Autodesk Inventor part; units mm, degrees
ref_plane "YZ Plane" through (0, 0, 0) normal (1, 0, 0) x (0, 1, 0)
ref_plane "XZ Plane" through (0, 0, 0) normal (0, 1, 0) x (-1, 0, 0)
ref_plane "XY Plane" through (0, 0, 0) normal (0, 0, 1) x (1, 0, 0)
sketch "Sketch4" plane through (0, 0, 0) normal (0, 0, 1) x (1, 0, 0)
  line L0 (0, 0) -> (26.5, 0)
  line L1 (26.5, 0) -> (26.5, 20.75)
  line L2 (0, 20.75) -> (0, 0)
  arc A0 (26.5, 20.75) -> (0, 20.75) centre (13.25, 20.75) ccw
  line L3 (-1.1061, 34) -> (25.3939, 34) construction
  dimension "d70" = 26.5
  dimension "d71" = 34
extrude "Plate3" add sketch "Sketch4" along normal blind 3
sketch "Sketch5" plane through (26.5, 3, 0) normal (0, -1, 0) x (1, 0, 0)
  line L0 (-26.5, 0) -> (0, 0)
  line L1 (0, 0) -> (0, 34)
  line L2 (0, 34) -> (-26.5, 34)
  line L3 (-26.5, 34) -> (-26.5, 0)
edge flange "Flange2" height 34 angle 90 thickness 3 bend radius 3 thickness toward (0, -1, 0) relief tear relief width 3 relief depth 1.5 edges at (13.25, 0, 3) wall of the first edge with corners at (0, 3, 0) (26.5, 3, 0) (26.5, 3, 34) (0, 3, 34)
bend "Bend2"
corner "Corner2"
sketch "Sketch8" plane through (0, 3, 3) normal (0, 0, 1) x (1, 0, 0)
  line L0 (26.5, 3) -> (0, 3)
  line L1 (13.25, 3) -> (13.25, 35.5458) construction
  line L2 (0, -3) -> (26.5, -3)
  point P0 (13.25, 17.75)
  point P1 (13.25, -3)
  dimension "d72" = 20.75
hole "Hole3" at (13.25, 20.75, 3) direction (0, 0, -1) diameter 8 end through all
sketch "Sketch11" plane through (0, 3, 34) normal (0, 1, 0) x (1, 0, 0)
  line L0 (0, 0) -> (26.5, 0)
  line L1 (13.25, 0) -> (13.25, 41.3955) construction
  point P0 (0, 34)
  point P1 (13.25, 15.2)
  dimension "d81" = 15.2
hole "Hole5" at (13.25, 3, 18.8) direction (0, -1, 0) diameter 6.9 end through all
sketch "Sketch12" plane through (0, 3, 34) normal (0, 1, 0) x (1, 0, 0)
  circle A0 centre (13.25, 15.2) radius 3.45
  circle A1 centre (13.25, 15.2) radius 10.6631 construction
  line L0 (0, 0) -> (26.5, 0)
  point P0 (0, 34)
  point P1 (21.25, 8.15)
  point P2 (5.25, 8.15)
  point P3 (5.25, 22.25)
  point P4 (21.25, 22.25)
  dimension "d89" = 16
  dimension "d90" = 8.15
hole "Hole6" at (21.25, 3, 25.85) at (5.25, 3, 25.85) at (5.25, 3, 11.75) at (21.25, 3, 11.75) direction (0, -1, 0) diameter 3.3 end through all
sketch "Sketch13" plane through (0, 0, 0) normal (0, 0, -1) x (-1, 0, 0)
  circle A0 centre (-13.25, 20.75) radius 4
  circle A1 centre (-13.25, 20.75) radius 8.5 construction
  point P0 (0, 0)
  point P1 (-21.75, 20.75)
  point P2 (-4.75, 20.75)
  dimension "d98" = 17
hole "Hole7" at (21.75, 20.75, 0) at (4.75, 20.75, 0) direction (0, 0, 1) diameter 3 end through all counterbore diameter 6 counterbore depth 2
equation "\"d27\" = Thickness"
equation "\"d28\" = BendReliefWidth"
equation "\"d29\" = BendReliefDepth"
equation "\"d30\" = MinimumRemnant"
equation "\"d31\" = TransitionRadius"
equation "\"d34\" = BendRadius"
equation "\"d35\" = CornerReliefSize"
equation "\"d36\" = GapSize"
equation "\"d37\" = JacobiRadiusSize"
equation "\"BendRadius\" = Thickness"
equation "\"BendReliefWidth\" = Thickness"
equation "\"BendReliefDepth\" = 0.5 * Thickness"
equation "\"CornerReliefSize\" = 4 * Thickness"
equation "\"MinimumRemnant\" = 2 * Thickness"
equation "\"TransitionRadius\" = BendRadius"
equation "\"JacobiRadiusSize\" = BendRadius"
equation "\"GapSize\" = Thickness"
properties part number "JGA25-370-bracket" material "Aluminum 6061"
The listing builds one solid part. Answer for the finished solid, in the listing's coordinates (mm). A direction names the side the tool comes from. Round coordinates to 2 decimals unless told otherwise and drop trailing zeros. Order: outer loops, then holes, each group sorted by start corner. A loop starts at its lowest first (then second) coordinate and runs counter-clockwise, first axis right, second up. Notation, with made-up numbers: (-8.5, 61) -> (47.5, 61) arc R24 ccw to (47.5, 73) -> close; hole circle Ø3 at (29, -6). An arc over 180 degrees is marked (long way). Put each result on its own line as item: value.
Q1. Determine the mould class of faces 1 (the cylindrical face through (13.098, 1.479, 15.353)), 2 (the flat face through (16, 17, 3)), 3 (the flat face through (0, 2.6, 13.3)), 4 (the cylindrical face through (20.135, 1.479, 24.634)) for opening direction Z: pulls with the +Z half, pulls with the -Z half, needs draft (parallel to the pull), parting line crosses it, or undercut.
Results list:
face 1: undercut
face 2: pulls with the +Z half
face 3: needs draft
face 4: undercut
Q2. Consider line 1 along X through (y, z) = (1.95, 11.75); line 2 along X through (y, z) = (20.75, 2.5); line 3 along Z through (x, y) = (21.25, 2.05). Determine where each line is inside the solid, lowest interval first.
Results list:
line 1: 0 to 3.6, 6.9 to 19.6, 22.9 to 26.5
line 2: 0 to 3.25, 6.25 to 9.25, 17.25 to 20.25, 23.25 to 26.5
line 3: 1.48 to 10.1, 13.4 to 24.2, 27.5 to 34
Q3. Which of the six approach directions +Z, -Z, +X, -X, +Y, -Y give full straight-line access (tool end or side, diameter ignored) to faces 5 (the flat face through (13, 3, 23)), 6 (the flat face through (13, 0, 23)), 7 (the cylindrical face through (23.575, 18.369, 1.014))?
Results list:
face 5: +Z, +X, -X, +Y
face 6: +Z, -Z, +X, -X, -Y
face 7: -Z
Q4. Section A-A, the plane x = 13.25 is taken. Write down the section's boundary in (y, z).
Results list:
outline: (0, 6) arc R6 ccw to (6, 0) -> (16.75, 0) -> (16.75, 3) -> (6, 3) arc R3 cw to (3, 6) -> (3, 15.35) -> (0, 15.35) -> close; (0, 22.25) -> (3, 22.25) -> (3, 34) -> (0, 34) -> close; (24.75, 0) -> (34, 0) -> (34, 3) -> (24.75, 3) -> close
Q5. Section D-D, the plane z = 11.75 is taken. Write down the section's boundary in (x, y).
Results list:
outline: (0, 0) -> (3.6, 0) -> (3.6, 3) -> (0, 3) -> close; (6.9, 0) -> (19.6, 0) -> (19.6, 3) -> (6.9, 3) -> close; (22.9, 0) -> (26.5, 0) -> (26.5, 3) -> (22.9, 3) -> close
Q6. Each of these flat-tipped pins is pushed along its axis until it touches: P1, Ø3, axis at x = 17, y = 27, coming from the +Z side; P2, Ø4.5, axis at x = 21.25, z = 25.85, coming from the +Y side; P3, Ø1, axis at x = 4.5, y = 4, coming from the -Z side. Where does it stop, or does it pass through?
Results list:
P1: z = 3
P2: y = 3
P3: z = 0.19
Q7. Section C-C, the plane y = 23 is taken. Write down the section's boundary in (x, z).
Results list:
outline: (0.19, 0) -> (2.77, 0) -> (2.77, 2) -> (6.73, 2) -> (6.73, 0) -> (9.94, 0) -> (9.94, 3) -> (0.19, 3) -> close; (16.56, 0) -> (19.77, 0) -> (19.77, 2) -> (23.73, 2) -> (23.73, 0) -> (26.31, 0) -> (26.31, 3) -> (16.56, 3) -> close
Q8. Section B-B, the plane z = 18.8 is taken. Write down the section's boundary in (x, y), and give its area (3 significant figures).
Results list:
outline: (0, 0) -> (9.8, 0) -> (9.8, 3) -> (0, 3) -> close; (16.7, 0) -> (26.5, 0) -> (26.5, 3) -> (16.7, 3) -> close
area: 58.8 mm^2
